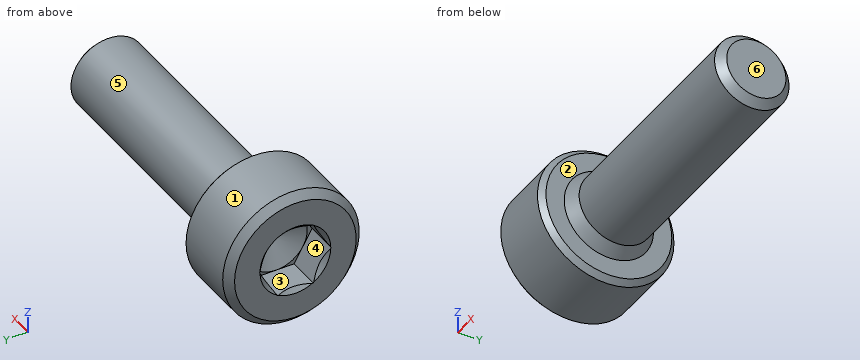
Autodesk Inventor part; units mm, degrees
ref_plane "ANBAU_XY" through (0, 0, 0) normal (-1, 0, 0) x (0, 0, -1)
ref_plane "ANBAU_YZ" through (0, 0, 0) normal (0, 0, -1) x (0, -1, 0)
ref_plane "ANBAU_ZX" through (0, 0, 0) normal (0, -1, 0) x (-1, 0, 0)
sketch "Sketch_1" plane through (0, 0, 0) normal (0, 0, 1) x (1, 0, 0)
  line L0 (10, 0) -> (-3, 0)
  line L1 (-3, 0) -> (-3, 2.75)
  line L2 (-3, 2.75) -> (0, 2.75)
  line L3 (0, 2.75) -> (0, 1.8)
  line L4 (0, 1.8) -> (0.51, 1.5)
  line L5 (0.51, 1.5) -> (9.6935, 1.5)
  line L6 (9.6935, 1.5) -> (10, 1.1935)
  line L7 (10, 1.1935) -> (10, 0)
  line L8 (10, 0) -> (-3, 0)
revolve "Revolution1" add sketch "Sketch_1" angle 360 about axis through (10, 0, 0) along (1, 0, 0)
thread "Thread1"
sketch "Sketch_6" plane through (0, 0, 0) normal (0, 0, 1) x (1, 0, 0)
  line L0 (0, 0) -> (-3, 0)
  line L1 (-3, 3.3) -> (-3, 2.45)
  line L2 (-3, 2.45) -> (-2.7, 2.75)
  line L3 (-2.7, 2.75) -> (-0.215, 2.75)
  line L4 (-0.215, 2.75) -> (0, 2.535)
  line L5 (0, 2.535) -> (0, 3.3)
  line L6 (0, 3.3) -> (-3, 3.3)
revolve "Revolution2" cut sketch "Sketch_6" angle 360 about axis through (0, 0, 0) along (1, 0, 0)
sketch "Sketch3" plane through (-3, 0, 0) normal (-1, 0, 0) x (0, 0, 1)
  point P0 (0, 0)
hole "Hole1" at (-3, 0, 0) direction (1, 0, 0) diameter 2.5 depth 1.3 tip angle 120 countersink diameter 2.85 countersink angle 90
sketch "Sketch_2" plane through (-3, 0, 0) normal (1, 0, 0) x (0, 0, -1)
  line L0 (-1.25, -0.7217) -> (0, -1.4434)
  line L1 (0, -1.4434) -> (1.25, -0.7217)
  line L2 (1.25, -0.7217) -> (1.25, 0.7217)
  line L3 (1.25, 0.7217) -> (0, 1.4434)
  line L4 (0, 1.4434) -> (-1.25, 0.7217)
  line L5 (-1.25, 0.7217) -> (-1.25, -0.7217)
extrude "Extrusion1" cut sketch "Sketch_2" along normal mid plane 2.6
ref_plane "ANBAU_XY" through (0, 0, 0) normal (-1, 0, 0) x (0, 0, -1)
ref_plane "ANBAU_YZ" through (0, 0, 0) normal (0, 0, -1) x (0, -1, 0)
ref_plane "ANBAU_ZX" through (0, 0, 0) normal (0, -1, 0) x (-1, 0, 0)
ref_plane "IP1_XY" through (0, 0, 0) normal (1, 0, 0) x (0, 0, -1)
ref_plane "IP1_YZ" through (0, 0, 0) normal (0, 0, -1) x (0, 1, 0)
ref_plane "IP1_ZX" through (0, 0, 0) normal (0, 1, 0) x (1, 0, 0)
ref_plane "IP2_XY" through (-3, 0, 0) normal (1, 0, 0) x (0, 0, -1)
ref_plane "IP2_YZ" through (-3, 0, 0) normal (0, 0, -1) x (0, 1, 0)
ref_plane "IP2_ZX" through (-3, 0, 0) normal (0, 1, 0) x (1, 0, 0)
ref_plane "IP3_XY" through (10, 0, 0) normal (1, 0, 0) x (0, 0, -1)
ref_plane "IP3_YZ" through (10, 0, 0) normal (0, 0, -1) x (0, 1, 0)
ref_plane "IP3_ZX" through (10, 0, 0) normal (0, 1, 0) x (1, 0, 0)
properties part number "ISO-4762 M3x10"
Geometry: final body of the model. Coordinates: model frame, mm. Face numbers are marked on the shaded views. A direction names the side the tool comes from. Round coordinates to 2 decimals unless told otherwise and drop trailing zeros. Order: outer loops, then holes, each group sorted by start corner. A loop starts at its lowest first (then second) coordinate and runs counter-clockwise, first axis right, second up.
Q1. Pin query (flat end, axial travel): pin 1 (3 mm diameter, centred on x = 5.5, z = -0.5, fed in from -Y); pin 2 (1.2 mm diameter, centred on y = 0.5, z = -0.5, fed in from -X); pin 3 (1.5 mm diameter, centred on x = 7.5, z = -1.5, fed in from +Y). Return the tip coordinate at first contact, or that it passes through.
Result sheet:
pin 1: stops at y = -1.5
pin 2: stops at x = -2.88
pin 3: stops at y = 1.3
Q2. Material intervals for probe 1 along X at (y, z) = (-2.2, 0.25); probe 2 along Y at (x, z) = (-1.5, -0.55); probe 3 along Z at (x, y) = (8, 0.2), sorted ascending.
Result sheet:
probe 1: x = -3 to 0
probe 2: y = -2.69 to -0.72, 0.72 to 2.69
probe 3: z = -1.49 to 1.49
Q3. Section A-A, the plane x = 4.25. Output: boundary loops of the cut face in (y, z).
Result sheet:
outline: circle Ø3 at (0, 0)
Q4. Mould query, pull axis Y, two halves, no side actions, for the marked faces 3, 4, 5 and 6. Classes: released by +Y, released by -Y, zero draft, split by the parting line, or undercut.
Result sheet:
face 3: undercut
face 4: undercut
face 5: split by the parting line
face 6: zero draft
Q5. Section B-B, the plane x = -1.25. Output: boundary loops of the cut face in (y, z), and give its area (3 significant figures).
Result sheet:
outline: circle Ø5.5 at (0, 0); hole circle Ø0.94 at (0, 0)
area: 23.1 mm2
Q6. Access query for the marked faces 1 and 2. Directions: +Z, -Z, +X, -X, +Y, -Y. A direction counts if a zero-diameter tool reaches every point of the face in a straight line with its end or side. Return the directions, or none.
Result sheet:
face 1: +X, -X
face 2: +X
Q7. Section C-C, the plane x = 0.25. Output: boundary loops of the cut face in (y, z).
Result sheet:
outline: circle Ø3.31 at (0, 0)
